Geometry check sheet. Reference: the model listing, model coordinates, mm. A direction names the side the tool comes from. Give positions to 0.01 mm unless a question says otherwise; leave off trailing zeros. Order: outer loops, then holes, each group sorted by start corner. A loop starts at its lowest first (then second) coordinate and runs counter-clockwise, first axis right, second up. Notation, with made-up numbers: M -17,-22.75 L 33,-22.75 A9 cw 33,-14.75 Z; hole C 35.25,36.5 d5. An arc over 180 degrees is marked long. Use CSV: the item, a comma, the result in double quotes. Start each with the question number.
from build123d import *

# Parameters (mm, degrees)
SKETCH1_W           = 45
SKETCH1_H           = 20
BOSS_EXTRUDE1_DEPTH = 1.6
SKETCH2_R           = 8
BOSS_EXTRUDE2_DEPTH = 14
SKETCH3_R           = 6.4
CUT_EXTRUDE1_DEPTH  = 0.5
FILLET1_R           = 0.5


with BuildPart() as part:
    # Sketch1 → Boss-Extrude1 (new body)
    with BuildSketch(Plane(origin=(0, 0, 0), x_dir=(1, 0, 0), z_dir=(0, 1, 0))):
        with Locations((22.5, 10)):
            Rectangle(SKETCH1_W, SKETCH1_H)
    extrude(amount=BOSS_EXTRUDE1_DEPTH)

    # Sketch2 → Boss-Extrude2 (add)
    with BuildSketch(Plane(origin=(0, 1.6, 0), x_dir=(1, 0, 0), z_dir=(0, 1, 0))):
        with Locations((10, 10)):
            Circle(SKETCH2_R)
        with Locations((35, 10)):
            Circle(SKETCH2_R)
    extrude(amount=BOSS_EXTRUDE2_DEPTH)

    # Sketch3 → Cut-Extrude1 (cut)
    with BuildSketch(Plane(origin=(0, 15.6, 0), x_dir=(1, 0, 0), z_dir=(0, 1, 0))):
        with Locations((10, 10)):
            Circle(SKETCH3_R)
        with Locations((35, 10)):
            Circle(SKETCH3_R)
    extrude(amount=-CUT_EXTRUDE1_DEPTH, mode=Mode.SUBTRACT)

    # Fillet1
    fillet1_edges = [part.edges().sort_by_distance(p)[0] for p in [
        (2, 15.6, -10),
        (27, 15.6, -10),
    ]]
    fillet(fillet1_edges, radius=FILLET1_R)


solid = part.part
(1) Access from +Z, -Z, +X, -X, +Y, -Y to the whole of each face (thin tool, end or side, straight path). Record for faces 1 (the face through (35, 15.1, -10)), 2 (the face through (0, 1, -10)).
(2) Sectioned sample at D-D on x = 24. Record the cut outline in (y, z), then the cut area to 3 significant figures.
(3) Sectioned sample at A-A on z = -10. Record the cut outline in (x, y).
(4) Go/stop test with flat-tipped pins: P1, Ø5, axis at x = 30.5, y = 13.5, coming from the +Z side; P2, Ø7.5, axis at x = 10, z = -10, coming from the +Y side; P3, Ø1.5, axis at y = 3.5, z = -2.5, coming from the +X side; P4, Ø1, axis at x = 35.5, z = -15.5, coming from the -Y side. Record where each tip stops, or that it passes through.
(5) Thickness scan on line 1 (X direction, y = 9.75, z = -9.75); line 2 (X direction, y = 15.3, z = -10); line 3 (X direction, y = 15.45, z = -10). Record the ranges inside material, lowest first.
(6) Sectioned sample at C-C on y = 8.75. Record the cut outline in (x, z), then the cut area to 3 significant figures.
(7) Sectioned sample at B-B on x = 10. Record the cut outline in (y, z).
(8) Draft check along Z on faces 3 (the face through (22, 1, 0)), 4 (the face through (22, 1.6, -10)), 5 (the face through (28.606, 15.354, -10.281)). Enter one of: +Z half, -Z half, draft (parallel to the pull), parting line (faces both ways), or undercut.
Responses:
1,face 1,"+Y"
1,face 2,"+Z, -Z, -X, +Y, -Y"
2,outline,"M 0,-20 L 1.6,-20 L 1.6,0 L 0,0 Z"
2,area,"32.0 mm2"
3,outline,"M 0,0 L 45,0 L 45,1.6 L 43,1.6 L 43,15.1 A0.5 ccw 42.5,15.6 L 41.4,15.6 L 41.4,15.1 L 28.6,15.1 L 28.6,15.6 L 27.5,15.6 A0.5 ccw 27,15.1 L 27,1.6 L 18,1.6 L 18,15.1 A0.5 ccw 17.5,15.6 L 16.4,15.6 L 16.4,15.1 L 3.6,15.1 L 3.6,15.6 L 2.5,15.6 A0.5 ccw 2,15.1 L 2,1.6 L 0,1.6 Z"
4,P1,"z = -2.25"
4,P2,"y = 15.1"
4,P3,"x = 39.29"
4,P4,"y = 0"
5,line 1,"2 to 18, 27 to 43"
5,line 2,"2.04 to 3.6, 16.4 to 17.96, 27.04 to 28.6, 41.4 to 42.96"
5,line 3,"2.14 to 3.6, 16.4 to 17.86, 27.14 to 28.6, 41.4 to 42.86"
6,outline,"C 10,-10 d16; C 35,-10 d16"
6,area,"402 mm2"
7,outline,"M 0,-20 L 1.6,-20 L 1.6,-18 L 15.1,-18 A0.5 ccw 15.6,-17.5 L 15.6,-16.4 L 15.1,-16.4 L 15.1,-3.6 L 15.6,-3.6 L 15.6,-2.5 A0.5 ccw 15.1,-2 L 1.6,-2 L 1.6,0 L 0,0 Z"
8,face 3,"+Z half"
8,face 4,"draft"
8,face 5,"undercut"
